The drawing under review shows one solid part. Ordinate dimensions are in mm from its lowest x, y, z. A direction names the side the tool comes from. Give positions to 0.01 mm unless a question says otherwise; leave off trailing zeros. Loops run counter-clockwise (first coordinate to the right, second up) from the corner with the lowest first, then second, coordinate; pieces in that order, holes last. Notation, with made-up numbers: M -34.5,21.5 L -29.5,21.5 A18 cw -29.5,32.5 Z; hole C -13,23.25 d1. An arc over 180 degrees is marked long. Write item = value, one per line. Start each with the question number.
1. We need section D-D on y = 20.5. Give the boundary of the cut face in (x, z), then the cut area to 3 significant figures.
2. We need section A-A on x = 20.1. Give the boundary of the cut face in (y, z), then the cut area to 3 significant figures.
3. We need section B-B on x = 4.6. Give the boundary of the cut face in (y, z) (1 decimal), then the cut area to 3 significant figures.
4. Wall thickness on line 1 along X through (y, z) = (10, 45); line 2 along X through (y, z) = (34, 46); line 3 along Z through (x, y) = (27.85, 0.7) (1 decimal): over which ranges is each line inside the solid? List them lowest first. Write a range as from..to.
5. For the marked faces 1 and 2, list the 3-axis set-ups (+Z, -Z, +X, -X, +Y, -Y) from which the entire face can be reached by the end or side of a thin tool; tool diameter is ignored.
6. We need section C-C on x = 27.85. Give the boundary of the cut face in (y, z) (1 decimal).
7. For pin 1 (4 mm diameter, centred on x = 12.35, z = 6.58, fed in from -Y); pin 2 (6.5 mm diameter, centred on x = 13.5, z = 7, fed in from -Y); pin 3 (2 mm diameter, centred on x = 12.5, z = 24, fed in from +Y), all flat-tipped, find the tip position at first contact; note any pin that passes through.
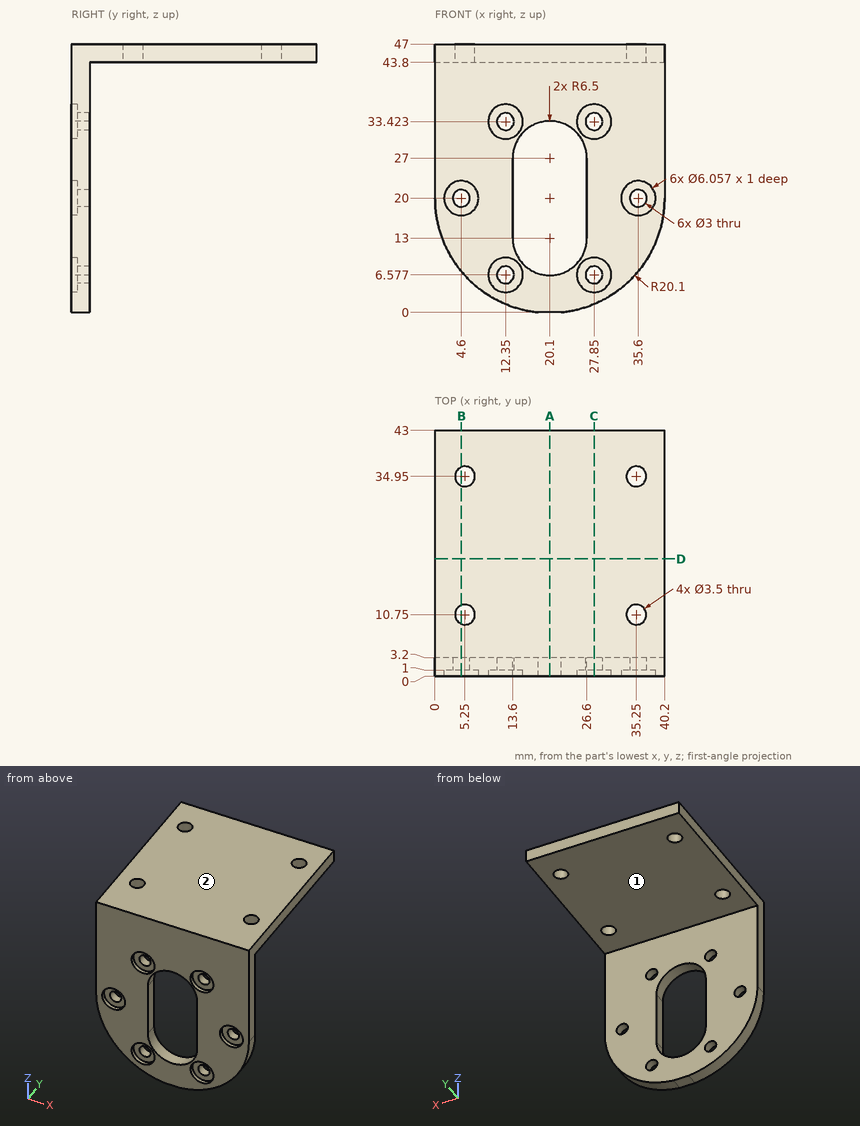
Final values:
q1.outline = M 0,43.8 L 40.2,43.8 L 40.2,47 L 0,47 Z
q1.area = 129 mm²
q2.outline = M 0,0 L 3.2,0 L 3.2,6.5 L 0,6.5 Z; M 0,33.5 L 3.2,33.5 L 3.2,43.8 L 43,43.8 L 43,47 L 0,47 Z
q2.area = 191 mm²
q3.outline = M 0,7.2 L 3.2,7.2 L 3.2,18.5 L 1,18.5 L 1,17 L 0,17 Z; M 0,23 L 1,23 L 1,21.5 L 3.2,21.5 L 3.2,43.8 L 9.1,43.8 L 9.1,47 L 0,47 Z; M 12.4,43.8 L 33.3,43.8 L 33.3,47 L 12.4,47 Z; M 36.6,43.8 L 43,43.8 L 43,47 L 36.6,47 Z
q3.area = 221 mm²
q4.line_1 = 0..3.67, 6.83..33.67, 36.83..40.2
q4.line_2 = 0..3.78, 6.72..33.78, 36.72..40.2
q4.line_3 = 1.5..3.5, 9.6..30.4, 36.5..47
q5.face_1 = -Z, +X, -X, +Y
q5.face_2 = +Z, +X, -X, +Y, -Y
q6.outline = M 0,1.5 L 3.2,1.5 L 3.2,5.1 L 1,5.1 L 1,3.5 L 0,3.5 Z; M 0,9.6 L 1,9.6 L 1,8.1 L 3.2,8.1 L 3.2,31.9 L 1,31.9 L 1,30.4 L 0,30.4 Z; M 0,36.5 L 1,36.5 L 1,34.9 L 3.2,34.9 L 3.2,43.8 L 43,43.8 L 43,47 L 0,47 Z
q7.pin_1 = 1
q7.pin_2 = 0
q7.pin_3 = 3.2
